Part model, mm, in its own coordinate system. A direction names the side the tool comes from. Coordinates: 2 decimals unless noted, no trailing zeros. Loops run counter-clockwise (first coordinate to the right, second up) from the corner with the lowest first, then second, coordinate; pieces in that order, holes last. Notation, with made-up numbers: (-12.75, 55.5) -> (3.25, 55.5) arc R19 cw to (3.25, 64.5) -> close; hole circle Ø5 at (-12, 58.25). An arc over 180 degrees is marked (long way). One line per item, written item: value. Start each with the question number.
from build123d import *

# Parameters (mm, degrees)
SKETCH1_W               = 104
SKETCH1_H               = 74
BOSS_EXTRUDE1_DEPTH     = 1
BOSS_EXTRUDE2_DEPTH     = 3
BOSS_EXTRUDE3_DEPTH     = 29.5
SKETCH3_W               = 104
SKETCH3_H               = 4
BOSS_EXTRUDE4_DEPTH     = 2
CUT_EXTRUDE1_DEPTH      = 11
CUT_EXTRUDE1_DEPTH_BACK = 11
CUT_EXTRUDE1_START      = -52
SKETCH5_W               = 104
SKETCH5_H               = 5
BOSS_EXTRUDE6_DEPTH     = 2
CUT_EXTRUDE2_START      = -32
CUT_EXTRUDE2_DEPTH      = 11
CUT_EXTRUDE3_START      = -83
CUT_EXTRUDE3_DEPTH      = 11


with BuildPart() as part:
    # Sketch1 → Boss-Extrude1 (new body)
    with BuildSketch(Plane.XY):
        with Locations((50, 37)):
            Rectangle(SKETCH1_W, SKETCH1_H)
    extrude(amount=BOSS_EXTRUDE1_DEPTH)

    # Sketch1<3> → Boss-Extrude2 (add)
    with BuildSketch(Plane.XY):
        Polygon((-2, 74), (-2, 0), (0, 0), (0, 72), (100, 72), (100, 0), (102, 0), (102, 74), align=None)
    extrude(amount=-BOSS_EXTRUDE2_DEPTH)

    # Sketch2 → Boss-Extrude3 (add)
    with BuildSketch(Plane(origin=(0, 0, -3), x_dir=(-1, 0, 0), z_dir=(0, 0, -1))):
        Polygon((-102, 74), (2, 74), (2, 70), (0, 70), (0, 72), (-100, 72), (-100, 70), (-102, 70), align=None)
    extrude(amount=BOSS_EXTRUDE3_DEPTH)

    # Sketch3 → Boss-Extrude4 (add)
    with BuildSketch(Plane.XZ):
        with Locations((50, -1)):
            Rectangle(SKETCH3_W, SKETCH3_H)
    extrude(amount=BOSS_EXTRUDE4_DEPTH)

    # Sketch4 → Cut-Extrude1 (cut, two sides: drawn at the far end of the back side and taken through both)
    with BuildSketch(Plane.ZY.offset(2).offset(CUT_EXTRUDE1_START - CUT_EXTRUDE1_DEPTH_BACK)):
        with BuildLine():
            Line((0, 0), (-2.4, 0))
            ThreePointArc((-2.4, 0), (-1.2, -1.2), (0, 0))
        make_face()
    extrude(amount=CUT_EXTRUDE1_DEPTH + CUT_EXTRUDE1_DEPTH_BACK, mode=Mode.SUBTRACT)

    # Sketch5 → Boss-Extrude6 (add)
    with BuildSketch(Plane(origin=(0, 0, -32.5), x_dir=(-1, 0, 0), z_dir=(0, 0, -1))):
        with Locations((-50, 71.5)):
            Rectangle(SKETCH5_W, SKETCH5_H)
    extrude(amount=BOSS_EXTRUDE6_DEPTH)

    # Sketch6 → Cut-Extrude2 (cut)
    with BuildSketch(Plane.ZY.offset(2).offset(CUT_EXTRUDE2_START)):
        with BuildLine():
            ThreePointArc((-32.5, 72.2), (-33.7, 71), (-32.5, 69.8))
            Line((-32.5, 69.8), (-32.5, 72.2))
        make_face()
    extrude(amount=CUT_EXTRUDE2_DEPTH, mode=Mode.SUBTRACT)

    # Sketch6<3> → Cut-Extrude3 (cut)
    with BuildSketch(Plane.ZY.offset(2).offset(CUT_EXTRUDE3_START)):
        with BuildLine():
            ThreePointArc((-32.5, 72.2), (-33.7, 71), (-32.5, 69.8))
            Line((-32.5, 69.8), (-32.5, 72.2))
        make_face()
    extrude(amount=CUT_EXTRUDE3_DEPTH, mode=Mode.SUBTRACT)


solid = part.part
1) Pin check, flat tips, straight feed: pin 1 Ø4 at (x, y) = (8.5, 52.5) entering from -Z; pin 2 Ø0.6 at (x, z) = (67, -33.5) entering from -Y; pin 3 Ø3 at (x, z) = (81, -16.5) entering from -Y. Stop position of each tip, or through.
2) Slice it at B-B (y = 59). Give the cut face in (x, z), then the cut area to 3 significant figures.
3) Pull direction Y, two halves, no side cores. Call faces 5 (the flat face through (26.6, -0.5, -3)), 6 (the flat face through (100, 47, -2)), 7 (the flat face through (49, -2, -1)), 8 (the flat face through (51, 74, -17)): +Y half, -Y half, draft (parallel to the pull), parting line (faces both ways), or undercut.
4) Slice it at C-C (z = -20). Give the cut face in (x, y), then the cut area to 3 significant figures.
5) Slice it at A-A (z = -1.2). Give the cut face in (x, y).
6) Probe line 1 (Y direction, x = 73, z = -1.5); line 2 (Y direction, x = 5.5, z = -19); line 3 (Z direction, x = 36.5, y = 28). List the from-to ranges inside material, lowest first. Write a range as from..to.
7) Tool access for faces 1 (the flat face through (49, 37, 1)), 2 (the flat face through (49.3, 0, -2.8)), 3 (the flat face through (51, 71, -32.5)), 4 (the cylindrical face through (24.6, 71, -33.7)): list every direction of +Z, -Z, +X, -X, +Y, -Y with a clear straight run to the whole face (end or side of a thin tool).
Check sheet entries:
1. pin 1: stops at z = 0
1. pin 2: stops at y = 69
1. pin 3: stops at y = 72
2. outline: (-2, -3) -> (0, -3) -> (0, 0) -> (100, 0) -> (100, -3) -> (102, -3) -> (102, 1) -> (-2, 1) -> close
2. area: 116 mm^2
3. face 5: draft
3. face 6: undercut
3. face 7: -Y half
3. face 8: +Y half
4. outline: (-2, 70) -> (0, 70) -> (0, 72) -> (100, 72) -> (100, 70) -> (102, 70) -> (102, 74) -> (-2, 74) -> close
4. area: 216 mm^2
5. outline: (-2, -2) -> (102, -2) -> (102, 74) -> (-2, 74) -> close; hole (0, 0) -> (39, 0) -> (39, -1.2) -> (61, -1.2) -> (61, 0) -> (100, 0) -> (100, 72) -> (0, 72) -> close
6. line 1: y = -2..0, 72..74
6. line 2: y = 72..74
6. line 3: z = 0..1
7. face 1: +Z, +X, -X, +Y, -Y
7. face 2: -Z
7. face 3: -Y
7. face 4: none
